Model file for the job. Use its own axes, mm. A direction names the side the tool comes from. Give positions to 0.01 mm unless a question says otherwise; leave off trailing zeros. Write each loop counter-clockwise with the first axis right and the second up, starting at its lowest first coordinate (ties: lowest second). Pieces come first, ordered by that corner, then holes.
```python
from build123d import *

# Parameters (mm, degrees)
F0_R     = 6.35
F1_DEPTH = 25.4
F2_SIZE  = 6.35
F3_W     = 63.5
F3_H     = 19.05
F4_DEPTH = 95.25
F6_DEPTH = 25.4
F7_R     = 6.35


with BuildPart() as f1:
    # F0 (on Top) → F1 (new body)
    with BuildSketch(Plane.XY):
        with BuildLine():
            Line((-13.251837, 83.219877), (-57.701837, 83.219877))
            ThreePointArc((-57.701837, 83.219877), (-68.927157, 78.570197), (-73.576837, 67.344877))
            Line((-73.576837, 67.344877), (-73.576837, 51.469877))
            Line((-73.576837, 51.469877), (2.623163, 51.469877))
            Line((2.623163, 51.469877), (2.623163, 67.344877))
            ThreePointArc((2.623163, 67.344877), (-2.026517, 78.570197), (-13.251837, 83.219877))
        make_face()
        with Locations((-57.701837, 67.344877)):
            Circle(F0_R, mode=Mode.SUBTRACT)
        with Locations((-13.251837, 67.344877)):
            Circle(F0_R, mode=Mode.SUBTRACT)
        Polygon((2.623163, 51.469877), (-73.576837, 51.469877), (-73.576837, 50.740071), (-73.576837, 32.419877), (2.623163, 32.419877), align=None)
        with BuildLine():
            Line((2.623163, -2.505123), (2.623163, 32.419877))
            Line((2.623163, 32.419877), (-73.576837, 32.419877))
            Line((-73.576837, 32.419877), (-73.576837, -2.505123))
            ThreePointArc((-73.576837, -2.505123), (-68.927157, -13.730443), (-57.701837, -18.380123))
            Line((-57.701837, -18.380123), (-13.251837, -18.380123))
            ThreePointArc((-13.251837, -18.380123), (-2.026517, -13.730443), (2.623163, -2.505123))
        make_face()
        with Locations((-57.701837, -2.505123)):
            Circle(F0_R, mode=Mode.SUBTRACT)
        with Locations((-13.251837, -2.505123)):
            Circle(F0_R, mode=Mode.SUBTRACT)
    extrude(amount=F1_DEPTH)

    # F2
    f2_edges = [f1.edges().sort_by_distance(p)[0] for p in [
        (-35.476837, 83.219877, 25.4),
    ]]
    chamfer(f2_edges, length=F2_SIZE)

    # F3 (on face) → F4 (join)
    with BuildSketch(Plane.XY.offset(25.4)):
        with Locations((-35.476837, 41.944877)):
            Rectangle(F3_W, F3_H)
    extrude(amount=F4_DEPTH)

    # F5 (on face) → F6 (cut)
    with BuildSketch(Plane.XZ.offset(-32.419877)):
        with BuildLine():
            ThreePointArc((-45.001837, 93.78757), (-35.476837, 95.25), (-25.951837, 93.78757))
            ThreePointArc((-25.951837, 93.78757), (-9.879169, 82.283553), (-3.726837, 63.5))
            Line((-3.726837, 63.5), (-3.726837, 120.65))
            Line((-3.726837, 120.65), (-67.226837, 120.65))
            Line((-67.226837, 120.65), (-67.226837, 63.5))
            ThreePointArc((-67.226837, 63.5), (-61.074506, 82.283553), (-45.001837, 93.78757))
        make_face()
        with BuildLine():
            ThreePointArc((-45.001837, 63.5), (-35.476837, 73.025), (-25.951837, 63.5))
            Line((-25.951837, 63.5), (-25.951837, 93.78757))
            ThreePointArc((-25.951837, 93.78757), (-35.476837, 95.25), (-45.001837, 93.78757))
            Line((-45.001837, 93.78757), (-45.001837, 63.5))
        make_face()
        with BuildLine():
            ThreePointArc((-45.001837, 63.5), (-35.476837, 53.975), (-25.951837, 63.5))
            ThreePointArc((-25.951837, 63.5), (-35.476837, 73.025), (-45.001837, 63.5))
        make_face()
    extrude(amount=-F6_DEPTH, mode=Mode.SUBTRACT)

    # F7
    f7_edges = [f1.edges().sort_by_distance(p)[0] for p in [
        (-35.476837, 51.469877, 25.4),
        (-35.476837, 32.419877, 25.4),
    ]]
    fillet(f7_edges, radius=F7_R)


solid = f1.part
```
1. Slice it at A-A, the plane z = 70. Write the cut outline in (x, y).
Calculated:
outline: (-66.55, 32.42) - (-45, 32.42) - (-45, 51.47) - (-66.55, 51.47) - close; (-25.95, 32.42) - (-4.4, 32.42) - (-4.4, 51.47) - (-25.95, 51.47) - close
2. Pull direction X, two halves, no side cores. Call faces 4 (the cylindrical face through (-35.686, 41.812, 53.977)), 5 (the cylindrical face through (-68.803, 78.693, 9.392)), 6 (the cylindrical face through (-9.84, 72.7, 12.52)), 7 (the flat face through (-35.79, -15.16, 22.27)): +X half, -X half, draft (parallel to the pull), parting line (faces both ways), or undercut.
Calculated:
face 4: undercut
face 5: -X half
face 6: undercut
face 7: draft
3. Which spindle directions (+Z, -Z, +X, -X, +Y, -Y) get a long thin tool onto all of the face, cutting with end or side? Do faces 1 (the flat face through (-29, 32.42, 55)), 2 (the cylindrical face through (-61.24, 41.812, 82.056)), 3 (the flat face through (-36, 67, 25.4)). Say none if no direction does.
Calculated:
face 1: +Z, +X, -X, -Y
face 2: +Z, -X, +Y, -Y
face 3: +Z, +X, -X, +Y
4. Probe probe 1 along X at (y, z) = (-4, 12); probe 2 along Z at (x, y) = (-36, 24.5); probe 3 along Y at (x, z) = (-30.5, 41). List the from-to ranges inside material, lowest first.
Calculated:
probe 1: x = -73.51 to -63.87, -51.53 to -19.42, -7.08 to 2.55
probe 2: z = 0 to 25.4
probe 3: y = 32.42 to 51.47
5. Slice it at D-D, the plane y = 10.5. Write the cut outline in (x, z), and give its area (3 significant figures).
Calculated:
outline: (-73.58, 0) - (2.62, 0) - (2.62, 19.05) - (-3.73, 25.4) - (-67.23, 25.4) - (-73.58, 19.05) - close
area: 1,900 mm2
6. Pin check, flat tips, straight feed: P1, Ø14.5, axis at x = -57.7, y = 67.34, coming from the +Z side; P2, Ø16, axis at y = 48, z = 46.5, coming from the +X side; P3, Ø16.5, axis at x = -57.7, y = -2.51, coming from the -Z side; P4, Ø8, axis at x = -11.5, z = 80.5, coming from the +Y side. Stop position of each tip, or through.
Calculated:
P1: stops at z = 25.4
P2: stops at x = -3.73
P3: stops at z = 0
P4: stops at y = 51.47
7. Slice it at B-B, the plane z = 14. Write the cut outline in (x, y) (3 decimals), and give its area (3 significant figures).
Calculated:
outline: (-73.577, -2.505) arc R15.875 ccw to (-57.702, -18.38) - (-13.252, -18.38) arc R15.875 ccw to (2.623, -2.505) - (2.623, 67.345) arc R15.875 ccw to (-13.252, 83.22) - (-57.702, 83.22) arc R15.875 ccw to (-73.577, 67.345) - close; hole circle Ø12.7 at (-57.702, -2.505); hole circle Ø12.7 at (-57.702, 67.345); hole circle Ø12.7 at (-13.252, -2.505); hole circle Ø12.7 at (-13.252, 67.345)
area: 7,020 mm2
8. Slice it at C-C, the plane x = -53. Write the cut outline in (y, z), and give its area (3 significant figures).
Calculated:
outline: (-18.38, 0) - (-6.77, 0) - (-6.77, 25.4) - (-12.03, 25.4) - (-18.38, 19.05) - close; (1.76, 0) - (63.08, 0) - (63.08, 25.4) - (57.82, 25.4) arc R6.35 cw to (51.47, 31.75) - (51.47, 89.98) - (32.42, 89.98) - (32.42, 31.75) arc R6.35 cw to (26.07, 25.4) - (1.76, 25.4) - close; (71.61, 0) - (83.22, 0) - (83.22, 19.05) - (76.87, 25.4) - (71.61, 25.4) - close
area: 3,350 mm2
